Autodesk Fusion 360 part; units mm, degrees
box "BoxPrimitive1" add length 650 width 1000 height 150 placed x (0, -1, 0) y (1, 0, 0) z (0, 0, 1) at (0, 0, 0)
sketch "Sketch3" plane through (0, 0, 150) normal (0, 0, 1) x (-1, 0, 0)
  line L0 (0, 650) -> (-1000, 650)
  line L1 (-1000, 650) -> (-1000, 0)
  line L2 (-1000, 0) -> (0, 0)
  line L3 (0, 0) -> (0, 650)
  line L4 (0, 0) -> (-150, 0)
  line L5 (-150, 0) -> (-150, 650)
  line L6 (-150, 650) -> (0, 650)
  line L7 (0, 650) -> (0, 0)
  line L8 (-150, 0) -> (-550, 0)
  line L9 (-550, 0) -> (-550, 400)
  line L10 (-550, 400) -> (-150, 400)
  line L11 (-150, 400) -> (-150, 0)
  line L12 (-550, 0) -> (-1000, 0)
  line L13 (-1000, 0) -> (-1000, 120)
  line L14 (-1000, 120) -> (-550, 120)
  line L15 (-550, 120) -> (-550, 0)
  line L16 (-800, 250) -> (-1000, 250)
  line L17 (-1000, 250) -> (-1000, 400)
  line L18 (-1000, 400) -> (-800, 400)
  arc A0 (-800, 250) -> (-800, 400) centre (-800, 325) ccw
  dimension "d6" = 150
  dimension "d7" = 400
  dimension "d8" = 400
  dimension "d9" = 120
  dimension "d10" = 150
  dimension "d11" = 200
extrude "Extrude1" add sketch "Sketch3" along normal blind 500 contours L0 L2 L3 L4 L5 L6 L7 L11
extrude "Extrude2" add sketch "Sketch3" along normal blind 300 contours L2 L5 L8 L9 L10 L11 L15 | L1 L2 L9 L12 L13 L14 L15
extrude "Extrude3" cut sketch "Sketch3" against normal blind 300 contours L1 L16 L17 L18 A0
fillet "Fillet1" radius 300 1 edges at (75, -650, 650)
chamfer "Chamfer1" distance 450 distance2 300 1 edges at (1000, -60, 450) measured on face at (283.3333, -173.3333, 450)
sketch "Sketch4" plane through (0, 0, 450) normal (0, 0, 1) x (-1, 0, 0)
  line L0 (-550, 120) -> (-550, 0)
  line L1 (-550, 0) -> (-150, 0)
  line L2 (-150, 0) -> (-150, 400)
  line L3 (-150, 400) -> (-550, 400)
  line L4 (-550, 400) -> (-550, 120)
  line L5 (-350, 0) -> (-470, 0)
  line L6 (-470, 0) -> (-470, 400)
  line L7 (-470, 400) -> (-350, 400)
  line L8 (-350, 400) -> (-350, 0)
  dimension "d22" = 120
  dimension "d23" = 400
revolve "Revolve1" cut sketch "Sketch4" angle 360 about axis through (350, -400, 450) along (0, 1, 0) contours L1 L3 L5 L6 L7 L8
For this review, take the finished solid that the model builds, in its own axes (mm). A direction names the side the tool comes from. Give positions to 0.01 mm unless a question says otherwise; leave off trailing zeros. Order: outer loops, then holes, each group sorted by start corner. A loop starts at its lowest first (then second) coordinate and runs counter-clockwise, first axis right, second up. Notation, with made-up numbers: (-32, 2) -> (-24, 2) arc R24 ccw to (-24, 13) -> close; hole circle Ø3 at (42.25, 23.5). An arc over 180 degrees is marked (long way). Write item = value, one per line.
1) We need section B-B, the plane z = 227. Give the boundary of the cut face in (x, y), and give its area (3 significant figures).
Findings:
outline = (0, -650) -> (150, -650) -> (150, -400) -> (550, -400) -> (550, -120) -> (884.5, -120) -> (884.5, 0) -> (0, 0) -> close
area = 298,000 mm^2
2) We need section C-C, the plane y = -325. Give the boundary of the cut face in (x, z), and give its area (3 significant figures).
Findings:
outline = (0, 0) -> (725, 0) -> (725, 150) -> (550, 150) -> (550, 450) -> (470, 450) arc R120 cw to (230, 450) -> (150, 450) -> (150, 650) -> (0, 650) -> close
area = 281,000 mm^2
3) To check wall thickness, follow L1, parallel to X at y = -152, z = 193; L2, parallel to X at y = -63.5, z = 559. State the ranges of each line that lie inside material, in increasing order. Write a range as from..to.
Findings:
L1 = 0..550
L2 = 0..150
4) Insertion check: pin 1 (10 mm diameter, centred on x = 526.5, y = -246, fed in from +Z); pin 2 (1.5 mm diameter, centred on x = 420, y = -167.5, fed in from +Z). Each pin has a flat end and moves straight along its axis. Give the tip position at first contact, or say it passes through.
Findings:
pin_1 = 450
pin_2 = 353.08
5) Draft analysis for pull direction Y (two halves, no side actions). For faces 1 (the face through (191, -203, 450)), 2 (the face through (76.05, -559.79, 564.45)), 3 (the face through (725.02, -323.35, 76.05)), state which applies: pulls with the +Y half, pulls with the -Y half, needs draft (parallel to the pull), parting line crosses it, or undercut.
Findings:
face_1 = needs draft
face_2 = pulls with the -Y half
face_3 = undercut
6) For faces 4 (the face through (678, -120, 231)), 5 (the face through (899, -250, 76)), 6 (the face through (382, 0, 176)), 7 (the face through (511, -203, 450)), 8 (the face through (347.36, -202.8, 330.03)), list the 3-axis set-ups (+Z, -Z, +X, -X, +Y, -Y) from which the entire face can be reached by the end or side of a thin tool; tool diameter is ignored.
Findings:
face_4 = +Z, +X, -Y
face_5 = +Z, -Z, +X
face_6 = +Z, -Z, +X, -X, +Y
face_7 = +Z, +X, +Y, -Y
face_8 = +Z, +Y, -Y
7) We need section D-D, the plane x = 350. Give the boundary of the cut face in (y, z).
Findings:
outline = (-650, 0) -> (0, 0) -> (0, 330) -> (-400, 330) -> (-400, 150) -> (-650, 150) -> close
8) We need section A-A, the plane x = 773. Give the boundary of the cut face in (y, z).
Findings:
outline = (-650, 0) -> (-394.97, 0) -> (-394.97, 150) -> (-650, 150) -> close; (-255.03, 0) -> (0, 0) -> (0, 301.33) -> (-120, 301.33) -> (-120, 150) -> (-255.03, 150) -> close
